Could you check a few things on this model? Use its own coordinates, in mm. A direction names the side the tool comes from. Round coordinates to 2 decimals unless told otherwise and drop trailing zeros. Loops run counter-clockwise (first coordinate to the right, second up) from the corner with the lowest first, then second, coordinate; pieces in that order, holes last. Notation, with made-up numbers: (-19, -11) -> (11, -11) arc R15 cw to (11, 3) -> close; hole circle Ø9 at (-36, -4). An arc over 180 degrees is marked (long way). Put each result on its own line as item: value. Start each with the question number.
1. Imagine slicing it at B-B, the plane z = -2. Please give me the cut outline in (x, y).
2. I'm going to push flat-ended pins straight in: P1, Ø1, axis at y = -46.5, z = -2, coming from the +X side; P2, Ø1.5, axis at x = 32, y = -46.5, coming from the +Z side; P3, Ø1.5, axis at y = -48, z = -2.5, coming from the -X side. Where does each tip first touch, or does it pass through?
3. Which directions (+Z, -Z, +X, -X, +Y, -Y) give clear straight access to the entire face, cutting with the end or side of a thin tool? Please do faces 1 (the flat face through (12.5, -48, -3)), 2 (the flat face through (31, -47, 5)), 3 (the flat face through (-23, -47, 0)).
4. Imagine slicing it at A-A, the plane y = -46. Please give me the cut outline in (x, z).
5. Imagine slicing it at C-C, the plane x = -26.5. Please give me the cut outline in (y, z).
6. I need wall thicknesses on line 1 (X direction, y = -48.45, z = 7); line 2 (X direction, y = -49.35, z = -2.5); line 3 (Z direction, x = 30, y = -46.3). Which ranges of each line are inside material? Lowest first, please. Write a range as [from, to].
```python
from build123d import *

# Parameters (mm, degrees)
SKETCH1_W           = 67.788084332
SKETCH1_H           = 5
BOSS_EXTRUDE1_DEPTH = 5
SKETCH2_W           = 57.788084332
SKETCH2_H           = 5
BOSS_EXTRUDE2_DEPTH = 5
SKETCH3_W           = 25
SKETCH3_H           = 5
BOSS_EXTRUDE3_DEPTH = 5


with BuildPart() as part:
    # Sketch1 → Boss-Extrude1 (new body)
    with BuildSketch(Plane.XY):
        with Locations((0, -47.5)):
            Rectangle(SKETCH1_W, SKETCH1_H)
    extrude(amount=BOSS_EXTRUDE1_DEPTH)

    # Sketch2 → Boss-Extrude2 (add)
    with BuildSketch(Plane.XY.offset(5)):
        with Locations((0, -47.5)):
            Rectangle(SKETCH2_W, SKETCH2_H)
    extrude(amount=BOSS_EXTRUDE2_DEPTH)

    # Sketch3 → Boss-Extrude3 (add)
    with BuildSketch(Plane.XZ.offset(50)):
        with Locations((0, -2.5)):
            Rectangle(SKETCH3_W, SKETCH3_H)
    extrude(amount=-BOSS_EXTRUDE3_DEPTH)


solid = part.part
```
Entries:
1. outline: (-12.5, -50) -> (12.5, -50) -> (12.5, -45) -> (-12.5, -45) -> close
2. P1: x = 12.5
2. P2: z = 5
2. P3: x = -12.5
3. face 1: -Z, +X, +Y, -Y
3. face 2: +Z, +X, +Y, -Y
3. face 3: -Z, -X, +Y, -Y
4. outline: (-33.89, 0) -> (-12.5, 0) -> (-12.5, -5) -> (12.5, -5) -> (12.5, 0) -> (33.89, 0) -> (33.89, 5) -> (28.89, 5) -> (28.89, 10) -> (-28.89, 10) -> (-28.89, 5) -> (-33.89, 5) -> close
5. outline: (-50, 0) -> (-45, 0) -> (-45, 10) -> (-50, 10) -> close
6. line 1: [-28.89, 28.89]
6. line 2: [-12.5, 12.5]
6. line 3: [0, 5]
